The listing builds one solid part. Answer for the finished solid, in the listing's coordinates (mm). Face numbers are marked on the shaded views. A direction names the side the tool comes from. Coordinates: 2 decimals unless noted, no trailing zeros. Order: outer loops, then holes, each group sorted by start corner. A loop starts at its lowest first (then second) coordinate and runs counter-clockwise, first axis right, second up. Notation, with made-up numbers: (51, 52.5) -> (89, 52.5) arc R12 cw to (89, 73.5) -> close; hole circle Ø9 at (-38.5, 25.25). An arc over 180 degrees is marked (long way). Write each question's results on one line, items separated by ' | '. Start each with the question number.
(1) The part is cut by section B-B, the plane y = 9. Count the separate pieces of the cut face and the enclosed holes in it, then the cut area to 3 significant figures.
(2) The part is cut by section D-D, the plane x = -44.5. Give the vertices of the cut face in (y, z).
(3) Given pin 1 (3 mm diameter, centred on x = -22.5, y = 13, fed in from -Z); pin 2 (6 mm diameter, centred on x = 16, z = 37, fed in from -Y); pin 3 (7.5 mm diameter, centred on y = 18.5, z = 122, fed in from +X); pin 4 (4 mm diameter, centred on y = 21.5, z = 195, fed in from -X), each flat-ended and moving along its own axis, determine where each tip first touches the part or whether it passes through.
(4) Straight lines are drawn through the part: L1, parallel to Z at x = 31.75, y = 6.5; L2, parallel to X at y = 21, z = 163.5; L3, parallel to X at y = 8.5, z = 198.12. For each, find the intervals that lie inside material, in ascending order.
(5) The part is cut by section C-C, the plane x = 10. Give the vertices of the cut face in (y, z) (3 decimals), then the cut area to 3 significant figures.
(6) The part is cut by section A-A, the plane z = 7.62. Give the vertices of the cut face in (x, y), then the cut area to 3 significant figures.
(7) A tool of negligible diameter and unlimited length cuts with its end or side. For the marked faces 1, 2, 3, 4 and 5, from which of +Z, -Z, +X, -X, +Y, -Y can it reach the whole face along a straight path? Write none if from no direction.
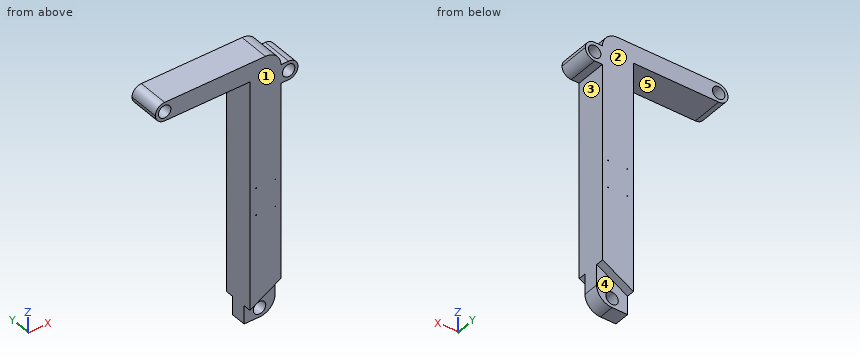
Autodesk Fusion 360 part; units mm, degrees
sketch "Sketch1" plane through (0, 0, 0) normal (0, 1, 0) x (1, 0, 0)
  line L0 (0, 0) -> (12.7, 0)
  line L1 (25.4, -12.7) -> (25.4, -218.44)
  line L2 (25.4, -218.44) -> (0, -218.44)
  line L3 (0, -218.44) -> (0, 0)
  line L4 (0, -218.44) -> (-77.47, -218.44)
  line L5 (-77.47, -218.44) -> (-77.47, -203.2)
  line L6 (-77.47, -203.2) -> (0, -203.2)
  line L7 (0, -203.2) -> (0, -218.44)
  line L8 (25.4, -205.74) -> (39.37, -205.74)
  line L9 (39.37, -205.74) -> (39.37, -190.5)
  line L10 (39.37, -190.5) -> (25.4, -190.5)
  line L11 (25.4, -190.5) -> (25.4, -205.74)
  circle A0 centre (-69.85, -210.82) radius 5.08
  circle A1 centre (31.75, -198.12) radius 5.08
  circle A2 centre (12.7, -7.62) radius 5.08
  arc A3 (25.4, -12.7) -> (12.7, 0) centre (12.7, -12.7) ccw
  point P0 (25.4, 0)
  dimension "d1" = 25.4
  dimension "d2" = 218.44
  dimension "d3" = 77.47
  dimension "d4" = 15.24
  dimension "d5" = 13.97
  dimension "d6" = 15.24
  dimension "d7" = 10.16
  dimension "d8" = 10.16
  dimension "d9" = 10.16
  dimension "d10" = 12.7
  dimension "d11" = 7.62
  dimension "d12" = 190.5
  dimension "d13" = 7.62
  dimension "d14" = 7.62
  dimension "d15" = 7.62
  dimension "d16" = 7.62
  dimension "d17" = 12.7
extrude "Extrude1" add sketch "Sketch1" along normal blind 25.4
sketch "Sketch2" plane through (0, 0, 0) normal (0, -1, 0) x (1, 0, 0)
  circle A0 centre (-69.85, 210.82) radius 5.08
  circle A1 centre (31.75, 198.12) radius 5.08
  circle A2 centre (12.7, 7.62) radius 5.08
  line L0 (39.37, 205.74) -> (25.4, 205.74)
  line L1 (25.4, 205.74) -> (25.4, 218.44)
  line L2 (25.4, 218.44) -> (-77.47, 218.44)
  line L3 (-77.47, 218.44) -> (-77.47, 203.2)
  line L4 (-77.47, 203.2) -> (0, 203.2)
  line L5 (0, 203.2) -> (0, 0)
  line L6 (0, 0) -> (12.7, 0)
  arc A3 (12.7, 0) -> (25.4, 12.7) centre (12.7, 12.7) ccw
  line L7 (25.4, 12.7) -> (25.4, 190.5)
  line L8 (25.4, 190.5) -> (39.37, 190.5)
  line L9 (39.37, 190.5) -> (39.37, 205.74)
  line L10 (0, 0) -> (0, 20.32)
  line L11 (25.4, 20.32) -> (0, 20.32)
  line L12 (25.4, 20.32) -> (25.4, 12.7)
  line L13 (0, 0) -> (12.7, 0)
  arc A4 (12.7, 0) -> (25.4, 12.7) centre (12.7, 12.7) ccw
extrude "Extrude2" cut sketch "Sketch2" against normal blind 6.3576 contours L5 L6 A3 L7 L10 L11 L12 L13 A4
sketch "Sketch3" plane through (0, 25.4, 0) normal (0, 1, 0) x (-1, 0, 0)
  circle A0 centre (69.85, 210.82) radius 5.08
  circle A1 centre (-31.75, 198.12) radius 5.08
  circle A2 centre (-12.7, 7.62) radius 5.08
  line L0 (-25.4, 205.74) -> (-39.37, 205.74)
  line L1 (-39.37, 205.74) -> (-39.37, 190.5)
  line L2 (-39.37, 190.5) -> (-25.4, 190.5)
  line L3 (-25.4, 190.5) -> (-25.4, 12.7)
  arc A3 (-25.4, 12.7) -> (-12.7, 0) centre (-12.7, 12.7) ccw
  line L4 (-12.7, 0) -> (0, 0)
  line L5 (0, 0) -> (0, 203.2)
  line L6 (0, 203.2) -> (77.47, 203.2)
  line L7 (77.47, 203.2) -> (77.47, 218.44)
  line L8 (77.47, 218.44) -> (-25.4, 218.44)
  line L9 (-25.4, 218.44) -> (-25.4, 205.74)
  line L10 (0, 0) -> (0, 20.32)
  line L11 (-25.4, 20.32) -> (0, 20.32)
  line L12 (0, 0) -> (-12.7, 0)
  line L13 (-25.4, 20.32) -> (-25.4, 12.7)
  arc A4 (-25.4, 12.7) -> (-12.7, 0) centre (-12.7, 12.7) ccw
extrude "Extrude3" cut sketch "Sketch3" against normal blind 6.3576 contours L3 A3 L4 L5 L10 L11 L12 L13 A4
extrude "Extrude4" add 1 faces at (16.9333, 2.1192, 20.32) along direction (0, 0, -1) blind 5.5118
sketch "Sketch4" plane through (0, 0, 0) normal (0, -1, 0) x (1, 0, 0)
  line L0 (25.4, 14.8082) -> (25.4, 190.5)
  line L1 (25.4, 190.5) -> (39.37, 190.5)
  line L2 (39.37, 190.5) -> (39.37, 205.74)
  line L3 (39.37, 205.74) -> (25.4, 205.74)
  line L4 (25.4, 205.74) -> (25.4, 218.44)
  line L5 (25.4, 218.44) -> (-77.47, 218.44)
  line L6 (-77.47, 218.44) -> (-77.47, 203.2)
  line L7 (-77.47, 203.2) -> (0, 203.2)
  line L8 (0, 203.2) -> (0, 14.8082)
  line L9 (0, 14.8082) -> (25.4, 14.8082)
  circle A0 centre (-69.85, 210.82) radius 5.08
  circle A1 centre (31.75, 198.12) radius 5.08
  line L10 (0, 14.8082) -> (25.4, 29.4729)
  line L11 (25.4, 29.4729) -> (0, 29.4729)
  line L12 (0, 14.8082) -> (0, 29.4729)
  dimension "d26" = 60
extrude "Extrude5" cut sketch "Sketch4" against normal blind 6.3576 contours L0 L9 L10
extrude "Extrude6" add 1 faces at (16.9333, 23.2808, 20.32) along direction (0, 0, -1) blind 5.5118
sketch "Sketch6" plane through (0, 25.4, 0) normal (0, 1, 0) x (-1, 0, 0)
  line L0 (0, 14.8082) -> (0, 203.2)
  line L1 (0, 203.2) -> (77.47, 203.2)
  line L2 (77.47, 203.2) -> (77.47, 218.44)
  line L3 (77.47, 218.44) -> (-25.4, 218.44)
  line L4 (-25.4, 218.44) -> (-25.4, 205.74)
  line L5 (-25.4, 205.74) -> (-39.37, 205.74)
  line L6 (-39.37, 205.74) -> (-39.37, 190.5)
  line L7 (-39.37, 190.5) -> (-25.4, 190.5)
  line L8 (-25.4, 190.5) -> (-25.4, 14.8082)
  line L9 (-25.4, 14.8082) -> (0, 14.8082)
  circle A0 centre (69.85, 210.82) radius 5.08
  circle A1 centre (-31.75, 198.12) radius 5.08
  line L10 (0, 14.8082) -> (-25.4, 29.4729)
  line L11 (-25.4, 29.4729) -> (0, 29.4729)
  line L12 (0, 14.8082) -> (0, 29.4729)
  dimension "d35" = 60
extrude "Extrude8" cut sketch "Sketch6" against normal blind 6.3576 contours L8 L9 L10
extrude "Extrude9" cut 2 faces at (16.9333, 4.2384, 24.5847) (16.9333, 21.1616, 24.5847) along direction (-0.5, 0, 0.866025) blind 0.254
fillet "Fillet1" radius 7.62 2 edges at (39.37, 12.7, 205.74) (39.37, 12.7, 190.5)
fillet "Fillet2" radius 7.62 2 edges at (-77.47, 12.7, 218.44) (-77.47, 12.7, 203.2)
fillet "Fillet3" radius 12.7 1 edges at (25.4, 12.7, 218.44)
sketch "Sketch7" plane through (0, 0, 0) normal (0, -1, 0) x (1, 0, 0)
  circle A0 centre (-69.85, 210.82) radius 5.08
  circle A1 centre (31.75, 198.12) radius 5.08
  arc A2 (25.4, 205.74) -> (12.7, 218.44) centre (12.7, 205.74) ccw
  line L0 (12.7, 218.44) -> (-69.85, 218.44)
  arc A3 (-69.85, 218.44) -> (-69.85, 203.2) centre (-69.85, 210.82) ccw
  line L1 (-69.85, 203.2) -> (0, 203.2)
  line L2 (0, 203.2) -> (0, 15.1015)
  line L3 (0, 15.1015) -> (25.273, 29.6929)
  line L4 (25.273, 29.6929) -> (25.4, 29.4729)
  line L5 (25.4, 29.4729) -> (25.4, 190.5)
  line L6 (25.4, 190.5) -> (31.75, 190.5)
  arc A4 (31.75, 190.5) -> (31.75, 205.74) centre (31.75, 198.12) ccw
  line L7 (31.75, 205.74) -> (25.4, 205.74)
  circle A5 centre (5.08, 91.3015) radius 0.3969
  circle A6 centre (20.7518, 91.3015) radius 0.3969
  circle A7 centre (5.08, 113.5265) radius 0.3969
  circle A8 centre (20.7518, 113.5265) radius 0.3969
  dimension "d46" = 0.7937
  dimension "d47" = 0.7937
  dimension "d48" = 0.7937
  dimension "d49" = 0.7937
  dimension "d50" = 15.6718
  dimension "d51" = 15.6718
  dimension "d52" = 22.225
  dimension "d53" = 5.08
  dimension "d54" = 76.2
hole "Hole1" at (5.08, 0, 113.5265) at (5.08, 0, 91.3015) at (20.7518, 0, 91.3015) at (20.7518, 0, 113.5265) direction (0, 1, 0) diameter 0.7937 depth 33.02 tip angle 118
Established:
1) separate pieces: 1 | enclosed holes: 7 | area: 6,580 mm^2
2) outline: (0, 203.2) -> (25.4, 203.2) -> (25.4, 218.44) -> (0, 218.44) -> close
3) pin 1: stops at z = 203.2 | pin 2: stops at y = 0 | pin 3: stops at x = 25.4 | pin 4: stops at x = 0
4) L1: z = 190.5 to 193.04, 203.2 to 205.74 | L2: x = 0 to 25.4 | L3: x = 0 to 26.67, 36.83 to 39.37
5) outline: (0, 20.875) -> (6.358, 20.875) -> (6.358, 11.923) -> (19.042, 11.923) -> (19.042, 20.875) -> (25.4, 20.875) -> (25.4, 218.44) -> (0, 218.44) -> close; (6.358, 0) -> (19.042, 0) -> (19.042, 3.317) -> (6.358, 3.317) -> close | area: 5,170 mm^2
6) outline: (0, 6.36) -> (7.62, 6.36) -> (7.62, 19.04) -> (0, 19.04) -> close; (17.78, 6.36) -> (24.34, 6.36) -> (24.34, 19.04) -> (17.78, 19.04) -> close | area: 180 mm^2
7) face 1: +Z, -Z, +X, -X, -Y | face 2: +Z, -Z, +X, -X, +Y | face 3: -Z, +X, +Y, -Y | face 4: -Z, +X, +Y | face 5: -Z, -X, +Y, -Y
